Autodesk Inventor part; units mm, degrees
ref_plane "YZ Plane" through (0, 0, 0) normal (1, 0, 0) x (0, 1, 0)
ref_plane "XZ Plane" through (0, 0, 0) normal (0, 1, 0) x (-1, 0, 0)
ref_plane "XY Plane" through (0, 0, 0) normal (0, 0, 1) x (1, 0, 0)
sketch "Sketch1" plane through (0, 0, 0) normal (0, 1, 0) x (-1, 0, 0)
  circle A0 centre (0, 0) radius 2.5
  dimension "d0" = 5
extrude "Extrusion1" add sketch "Sketch1" along normal blind 10
sketch "Sketch2" plane through (0, 10, 0) normal (0, 1, 0) x (1, 0, 0)
  circle A0 centre (0, 0) radius 2.5
  circle A1 centre (0, 0) radius 4.25
  dimension "d3" = 8.5
extrude "Extrusion2" add sketch "Sketch2" along normal blind 5 contours A0 | A1
sketch "Sketch3" plane through (0, 15, 0) normal (0, 1, 0) x (1, 0, 0)
  circle A0 centre (0, 0) radius 4.25
  line L0 (0, 2.3094) -> (2, 1.1547)
  line L1 (2, 1.1547) -> (2, -1.1547)
  line L2 (2, -1.1547) -> (0, -2.3094)
  line L3 (0, -2.3094) -> (-2, -1.1547)
  line L4 (-2, -1.1547) -> (-2, 1.1547)
  line L5 (-2, 1.1547) -> (0, 2.3094)
  dimension "d6" = 2
extrude "Extrusion3" cut sketch "Sketch3" against normal blind 3.2 contours L0 L1 L2 L3 L4 L5
thread "Thread1"
chamfer "Chamfer1" distance 0.25 angle 45 1 edges at (2.5, 0, 0)
properties part number "M5x10SHCS" material "Stainless Steel"
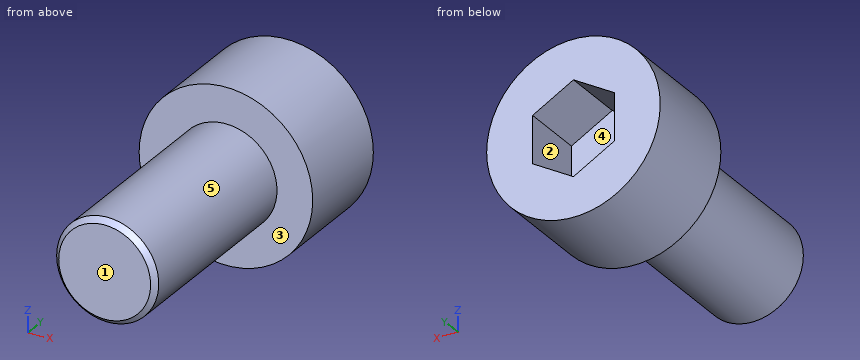
Model file for the job. Use its own axes, mm. Face numbers are marked on the shaded views. A direction names the side the tool comes from. Round coordinates to 2 decimals unless told otherwise and drop trailing zeros. Order: outer loops, then holes, each group sorted by start corner. A loop starts at its lowest first (then second) coordinate and runs counter-clockwise, first axis right, second up. Notation, with made-up numbers: M 13,-20.5 L 40,-20.5 A9 ccw 40,-12.5 Z; hole C 19,9.5 d6. An arc over 180 degrees is marked long. Write each question's results on one line, items separated by ' | '. Start each with the question number.
(1) Probe probe 1 along Y at (x, z) = (2.75, -1.75); probe 2 along X at (y, z) = (13, -2.25); probe 3 along Z at (x, y) = (-3.75, 13.75). List the from-to ranges inside material, lowest first. Write a range as from..to.
(2) Which spindle directions (+Z, -Z, +X, -X, +Y, -Y) get a long thin tool onto all of the face, cutting with end or side? Do the marked faces 1 and 2. Say none if no direction does.
(3) Saw through at C-C, the plane y = 1.5. Give the cut face in (x, z).
(4) Drop flat-ended pins along their axis: pin 1 (1.5 mm diameter, centred on y = 7, z = 1.5, fed in from +X); pin 2 (1 mm diameter, centred on y = 10.5, z = 2, fed in from +X); pin 3 (1 mm diameter, centred on x = -0.5, y = 9, fed in from +Z). Give the stop position or say it passes through.
(5) Saw through at A-A, the plane y = 12.25. Give the cut face in (x, z), then the cut area to 3 significant figures.
(6) Saw through at B-B, the plane z = 0. Give the cut face in (x, y).
(7) Saw through at D-D, the plane x = 3. Give the cut face in (y, z), then the cut area to 3 significant figures.
(8) Two-plate mould, pull along Z, no slides. Class the marked faces 3, 4 and 5: pulls with the +Z half, pulls with the -Z half, needs draft (parallel to the pull), parting line crosses it, or undercut.
Established:
1) probe 1: y = 10..15 | probe 2: x = -3.61..-0.1, 0.1..3.61 | probe 3: z = -2..2
2) face 1: +Z, -Z, +X, -X, -Y | face 2: +Y
3) outline: C 0,0 d5
4) pin 1: stops at x = 2.38 | pin 2: stops at x = 3.98 | pin 3: stops at z = 2.5
5) outline: C 0,0 d8.5; hole M -2,-1.15 L 0,-2.31 L 2,-1.15 L 2,1.15 L 0,2.31 L -2,1.15 Z | area: 42.9 mm^2
6) outline: M -4.25,10 L -2.5,10 L -2.5,0.25 L -2.25,0 L 2.25,0 L 2.5,0.25 L 2.5,10 L 4.25,10 L 4.25,15 L 2,15 L 2,11.8 L -2,11.8 L -2,15 L -4.25,15 Z
7) outline: M 10,-3.01 L 15,-3.01 L 15,3.01 L 10,3.01 Z | area: 30.1 mm^2
8) face 3: needs draft | face 4: undercut | face 5: parting line crosses it
